Input: part model. Units: mm. Frame: model coordinates. A direction names the side the tool comes from. Give positions to 0.01 mm unless a question says otherwise; leave off trailing zeros. Loops run counter-clockwise (first coordinate to the right, second up) from the corner with the lowest first, then second, coordinate; pieces in that order, holes last. Notation, with made-up numbers: (6.5, -39) -> (65.5, -39) arc R12 cw to (65.5, -19) -> close; hole circle Ø2 at (1, 57.25). An arc over 180 degrees is marked (long way). One line per question, with ' | ' between items.
from build123d import *

# Parameters (mm, degrees)
F0_R     = 12.45
F0_R_2   = 4.06
F1_DEPTH = 15.29


with BuildPart() as f1:
    # F0 (on Top) → F1 (new body)
    with BuildSketch(Plane.XY):
        Circle(F0_R)
        with BuildLine():
            ThreePointArc((-5.200227, -8.482932), (-8.147706, -5.711164), (-9.747939, -1.995039))
            ThreePointArc((-9.747939, -1.995039), (-7.860658, -2.357112), (-5.942674, -2.23766))
            ThreePointArc((-5.942674, -2.23766), (-5.197891, -3.647524), (-4.125369, -4.827404))
            ThreePointArc((-4.125369, -4.827404), (-4.893916, -6.587211), (-5.200227, -8.482932))
        make_face(mode=Mode.SUBTRACT)
        Circle(F0_R_2, mode=Mode.SUBTRACT)
        with BuildLine():
            ThreePointArc((6.460789, -7.56708), (2.91386, -9.513775), (-1.114884, -9.887342))
            ThreePointArc((-1.114884, -9.887342), (-0.187331, -8.204317), (0.291754, -6.343294))
            ThreePointArc((0.291754, -6.343294), (1.862765, -6.070635), (3.316325, -5.415209))
            ThreePointArc((3.316325, -5.415209), (4.752506, -6.689951), (6.460789, -7.56708))
        make_face(mode=Mode.SUBTRACT)
        with BuildLine():
            ThreePointArc((9.193215, 3.806219), (9.94857, -0.168673), (9.058903, -4.115674))
            ThreePointArc((9.058903, -4.115674), (7.744881, -2.713435), (6.122988, -1.682711))
            ThreePointArc((6.122988, -1.682711), (6.349143, -0.104335), (6.174971, 1.48062))
            ThreePointArc((6.174971, 1.48062), (7.831127, 2.452594), (9.193215, 3.806219))
        make_face(mode=Mode.SUBTRACT)
        with BuildLine():
            ThreePointArc((-9.674706, 2.32434), (-7.949419, 5.984082), (-4.909674, 8.65434))
            ThreePointArc((-4.909674, 8.65434), (-4.670823, 6.747542), (-3.964528, 4.960344))
            ThreePointArc((-3.964528, 4.960344), (-5.075238, 3.816341), (-5.865943, 2.43171))
            ThreePointArc((-5.865943, 2.43171), (-7.777113, 2.618831), (-9.674706, 2.32434))
        make_face(mode=Mode.SUBTRACT)
        with BuildLine():
            ThreePointArc((-0.77907, 9.919453), (3.234695, 9.40953), (6.713594, 7.343715))
            ThreePointArc((6.713594, 7.343715), (4.97393, 6.527322), (3.492461, 5.303321))
            ThreePointArc((3.492461, 5.303321), (2.061221, 6.006152), (0.500017, 6.330283))
            ThreePointArc((0.500017, 6.330283), (0.087396, 8.205737), (-0.77907, 9.919453))
        make_face(mode=Mode.SUBTRACT)
    extrude(amount=F1_DEPTH)


solid = f1.part
1. Section query B-B (z = 5.5). Output: boundary loops of the cut face in (x, y).
Determined:
outline: circle Ø24.9 at (0, 0); hole (-9.75, -2) arc R9.95 ccw to (-5.2, -8.48) arc R7.65 cw to (-4.13, -4.83) arc R6.35 cw to (-5.94, -2.24) arc R7.65 cw to start; hole (-9.67, 2.32) arc R7.65 cw to (-5.87, 2.43) arc R6.35 cw to (-3.96, 4.96) arc R7.65 cw to (-4.91, 8.65) arc R9.95 ccw to start; hole circle Ø8.12 at (0, 0); hole (-1.11, -9.89) arc R9.95 ccw to (6.46, -7.57) arc R7.65 cw to (3.32, -5.42) arc R6.35 cw to (0.29, -6.34) arc R7.65 cw to start; hole (-0.78, 9.92) arc R7.65 cw to (0.5, 6.33) arc R6.35 cw to (3.49, 5.3) arc R7.65 cw to (6.71, 7.34) arc R9.95 ccw to start; hole (6.12, -1.68) arc R7.65 cw to (9.06, -4.12) arc R9.95 ccw to (9.19, 3.81) arc R7.65 cw to (6.17, 1.48) arc R6.35 cw to start
2. Section query C-C (x = -3). Output: boundary loops of the cut face in (y, z).
Determined:
outline: (-12.08, 0) -> (-2.74, 0) -> (-2.74, 15.29) -> (-12.08, 15.29) -> close; (2.74, 0) -> (12.08, 0) -> (12.08, 15.29) -> (2.74, 15.29) -> close
3. Pull-direction query (Y, two-part tool) for faces 3 (the cylindrical face through (-9.18, 8.41, 7.54)), 4 (the flat face through (-3, 3, 0)), 5 (the cylindrical face through (2.968, -9.497, 7.538)); classes: pulls with the +Y half, pulls with the -Y half, needs draft (parallel to the pull), parting line crosses it, or undercut.
Determined:
face 3: parting line crosses it | face 4: needs draft | face 5: undercut
4. Ray query, line 1 along X through (y, z) = (5.75, 2.5); line 2 along Y through (x, z) = (-8.75, 2); line 3 along X through (y, z) = (1.5, 7.5). Return the intervals inside material, ascending. Write a range as from..to.
Determined:
line 1: x = -11.04..-8.12, -4.34..2.69, 3.95..11.04 | line 2: y = -8.86..-4.74, -2.25..2.53, 4.74..8.86 | line 3: x = -12.36..-3.77, 3.77..6.22, 9.84..12.36
5. Pin query (flat end, axial travel): P1, Ø6, axis at y = -8, z = 5.5, coming from the -X side; P2, Ø8, axis at x = 6, z = 4, coming from the -Y side; P3, Ø6, axis at x = 7, z = 6.5, coming from the +Y side; P4, Ø1, axis at x = -7, y = -2.5, coming from the +Z side. Return the tip coordinate at first contact, or that it passes through.
Determined:
P1: stops at x = -11.4 | P2: stops at y = -12.29 | P3: stops at y = 11.79 | P4: stops at z = 15.29
6. Section query D-D (x = 2). Output: boundary loops of the cut face in (y, z).
Determined:
outline: (-12.29, 0) -> (-9.75, 0) -> (-9.75, 15.29) -> (-12.29, 15.29) -> close; (-6.03, 0) -> (-3.53, 0) -> (-3.53, 15.29) -> (-6.03, 15.29) -> close; (3.53, 0) -> (6.03, 0) -> (6.03, 15.29) -> (3.53, 15.29) -> close; (9.75, 0) -> (12.29, 0) -> (12.29, 15.29) -> (9.75, 15.29) -> close
7. Reachability of faces 1 (the flat face through (-3, 3, 15.29)), 2 (the cylindrical face through (1.841, -6.077, 7.538)) from +Z, -Z, +X, -X, +Y, -Y: full face, straight path, thin tool, end or side. Return the list, or none.
Determined:
face 1: +Z, +X, -X, +Y, -Y | face 2: +Z, -Z
8. Section query A-A (y = 0). Output: boundary loops of the cut face in (x, z), then the cut area to 3 significant figures.
Determined:
outline: (-12.45, 0) -> (-4.06, 0) -> (-4.06, 15.29) -> (-12.45, 15.29) -> close; (4.06, 0) -> (6.35, 0) -> (6.35, 15.29) -> (4.06, 15.29) -> close; (9.95, 0) -> (12.45, 0) -> (12.45, 15.29) -> (9.95, 15.29) -> close | area: 202 mm2
